from build123d import *

# Parameters (mm, degrees)
SKETCH_1_R      = 5
SKETCH_1_R_2    = 1.8
SKETCH_1_R_3    = 10
SKETCH_1_R_4    = 1.6
EXTRUDE_1_DEPTH = 3


with BuildPart() as part:
    # 草图1 → 凸台-拉伸1 (new body)
    # profile 1 of 3: a face of its own
    with BuildSketch(Plane(origin=(0, 0, 0), x_dir=(1, 0, 0), z_dir=(0, 1, 0))):
        with Locations((0, 50)):
            Circle(SKETCH_1_R)
        with Locations(Location((0, 50, 0), (0, 0, 270))):
            Circle(SKETCH_1_R_2, mode=Mode.SUBTRACT)
    # profile 2 of 3: a face of its own
    with BuildSketch(Plane(origin=(0, 0, 0), x_dir=(1, 0, 0), z_dir=(0, 1, 0))):
        with BuildLine():
            ThreePointArc((5, 50), (-0.250313875, 45.006269634), (-4.974937186, 50.5))
            Line((-4.974937186, 50.5), (-9.949874371, 1))
            ThreePointArc((-9.949874371, 1), (0, 10), (9.949874371, 1))
            Line((9.949874371, 1), (4.974937186, 50.5))
            ThreePointArc((4.974937186, 50.5), (4.993730366, 50.250313875), (5, 50))
        make_face()
    # profile 3 of 3: a face of its own
    with BuildSketch(Plane(origin=(0, 0, 0), x_dir=(1, 0, 0), z_dir=(0, 1, 0))):
        Circle(SKETCH_1_R_3)
        with Locations(Location((7, 0, 0), (0, 0, 270))):
            Circle(SKETCH_1_R_4, mode=Mode.SUBTRACT)
        with Locations(Location((0, 7, 0), (0, 0, 270))):
            Circle(SKETCH_1_R_4, mode=Mode.SUBTRACT)
        with Locations(Location((0, 0, 0), (0, 0, 270))):
            Circle(SKETCH_1_R_4, mode=Mode.SUBTRACT)
        with Locations(Location((0, -7, 0), (0, 0, 270))):
            Circle(SKETCH_1_R_4, mode=Mode.SUBTRACT)
        with Locations(Location((-7, 0, 0), (0, 0, 270))):
            Circle(SKETCH_1_R_4, mode=Mode.SUBTRACT)
    extrude(amount=EXTRUDE_1_DEPTH)


solid = part.part
Here's how the part is built. I have some questions about the finished solid (model axes, mm). Round coordinates to 2 decimals unless told otherwise and drop trailing zeros. Order: outer loops, then holes, each group sorted by start corner. A loop starts at its lowest first (then second) coordinate and runs counter-clockwise, first axis right, second up. Notation, with made-up numbers: M 22,-4.75 L 80,-4.75 A24 ccw 80,7.25 Z; hole C 35,-40 d1. An arc over 180 degrees is marked long. Return JSON: item names as keys, results as strings. Group by question number.
1. Please list where these lines run through material, in increasing order: probe 1 along X at (y, z) = (2.1, 0); probe 2 along X at (y, z) = (2.1, 7); probe 3 along X at (y, z) = (2.15, -13.5).
2. If we section it at C-C on x = 0: List the corners of the cut face in (y, z) for me, then the cut area to 3 significant figures.
3. If we mould it in two halves opening along Z, with no side actions, what happens to faces 1 (the face through (5.44, 1.48, -0.35)), 2 (the face through (0, 0, -23)), 3 (the face through (0, 1, -55))? For each: pulls with the +Z half, pulls with the -Z half, needs draft (parallel to the pull), parting line crosses it, or undercut.
4. If we section it at A-A on z = 0: List the corners of the cut face in (x, y) for me.
5. If we section it at D-D on z = 7: List the corners of the cut face in (x, y) for me.
6. I'm going to push flat-ended pins straight in: pin 1 Ø1 at (y, z) = (0.5, -31.5) entering from -X; pin 2 Ø1 at (x, y) = (8, 0.5) entering from +Z. Where does each tip first touch, or does it pass through?
7. If we section it at B-B on y = 0.6: List the corners of the cut face in (x, z) for me.
Reply:
{
 "1": {"probe 1": "-10 to -8.6, -5.4 to -1.6, 1.6 to 5.4, 8.6 to 10", "probe 2": "-7.14 to -1.6, 1.6 to 7.14", "probe 3": "-8.69 to 8.69"},
 "2": {"outline": "M 0,-55 L 3,-55 L 3,-51.8 L 0,-51.8 Z; M 0,-48.2 L 3,-48.2 L 3,-8.6 L 0,-8.6 Z; M 0,-5.4 L 3,-5.4 L 3,-1.6 L 0,-1.6 Z; M 0,1.6 L 3,1.6 L 3,5.4 L 0,5.4 Z; M 0,8.6 L 3,8.6 L 3,10 L 0,10 Z", "area": "155 mm^2"},
 "3": {"face 1": "undercut", "face 2": "needs draft", "face 3": "pulls with the -Z half"},
 "4": {"outline": "M -10,0 L -8.6,0 L -8.6,3 L -10,3 Z; M -5.4,0 L -1.6,0 L -1.6,3 L -5.4,3 Z; M 1.6,0 L 5.4,0 L 5.4,3 L 1.6,3 Z; M 8.6,0 L 10,0 L 10,3 L 8.6,3 Z"},
 "5": {"outline": "M -7.14,0 L -1.6,0 L -1.6,3 L -7.14,3 Z; M 1.6,0 L 7.14,0 L 7.14,3 L 1.6,3 Z"},
 "6": {"pin 1": "x = -6.93", "pin 2": "z = 6.61"},
 "7": {"outline": "M -9.95,-1 L -4.97,-50.5 A5 ccw 4.97,-50.5 L 9.95,-1 A10 ccw long Z; hole C -7,0 d3.2; hole C 0,-50 d3.6; hole C 0,-7 d3.2; hole C 0,0 d3.2; hole C 0,7 d3.2; hole C 7,0 d3.2"}
}
